The listing builds one solid part. Answer for the finished solid, in the listing's coordinates (mm). Face numbers are marked on the shaded views. A direction names the side the tool comes from. Give positions to 0.01 mm unless a question says otherwise; leave off trailing zeros. Write each loop counter-clockwise with the first axis right and the second up, starting at its lowest first coordinate (ties: lowest second). Pieces come first, ordered by that corner, then holes. Notation, with made-up numbers: (11, 47.25) - (22, 47.25) arc R20 cw to (22, 70.25) - close; hole circle Ø3 at (-14.75, 20.5). An arc over 180 degrees is marked (long way). Answer in a Markdown table with one row per item. Add a question column.
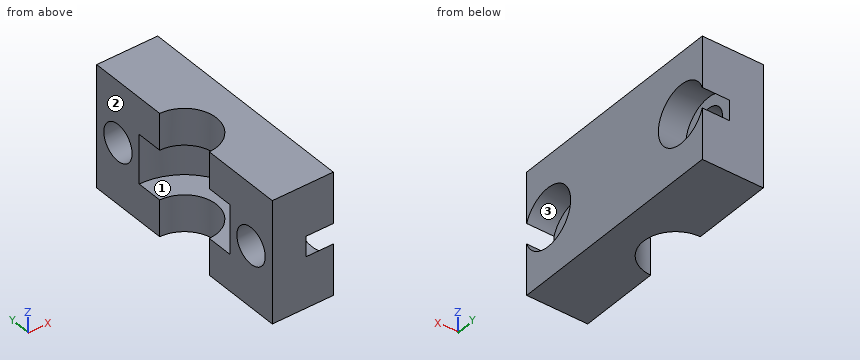
from build123d import *

# Parameters (mm, degrees)
EXTRUDE_1_DEPTH     = 2.7
SKETCH_1_4_W        = 3.35
SKETCH_1_4_H        = 12.4
EXTRUDE_2_DEPTH     = 2
EXTRUDE_START       = 2.7
SKETCH_1_5_W        = 3.35
SKETCH_1_5_H        = 12.4
EXTRUDE_3_DEPTH     = 2
SKETCH_2_R          = 1.75
CUT_EXTRUDE_1_DEPTH = 10.723810981
SKETCH_4_R          = 1
CUT_EXTRUDE_2_DEPTH = 9.470684742
SKETCH_4_3_R        = 1.6
SKETCH_4_3_R_2      = 1
CUT_EXTRUDE_3_DEPTH = 1.5


with BuildPart() as part:
    # 草图1 → 凸台-拉伸1 (new body)
    with BuildSketch(Plane.XY):
        with BuildLine():
            Line((3.35, 6.2), (0, 6.2))
            Line((0, 6.2), (0, 3.2))
            ThreePointArc((0, 3.2), (2.2627417, 2.2627417), (3.2, 0))
            ThreePointArc((3.2, 0), (2.2627417, -2.2627417), (0, -3.2))
            Line((0, -3.2), (0, -6.2))
            Line((0, -6.2), (3.35, -6.2))
            Line((3.35, -6.2), (3.35, 6.2))
        make_face()
    extrude(amount=EXTRUDE_1_DEPTH)

    # 草图1<4> → 凸台-拉伸2 (add)
    with BuildSketch(Plane.XY):
        with Locations((1.675, 0)):
            Rectangle(SKETCH_1_4_W, SKETCH_1_4_H)
    extrude(amount=-EXTRUDE_2_DEPTH)

    # 草图1<5> → 凸台-拉伸3 (add)
    with BuildSketch(Plane.XY.offset(EXTRUDE_START)):
        with Locations((1.675, 0)):
            Rectangle(SKETCH_1_5_W, SKETCH_1_5_H)
    extrude(amount=EXTRUDE_3_DEPTH)

    # 草图2 → 切除-拉伸1 (cut, through all)
    with BuildSketch(Plane.XY.offset(4.7)):
        Circle(SKETCH_2_R)
    extrude(amount=-CUT_EXTRUDE_1_DEPTH, mode=Mode.SUBTRACT)

    # 草图4 → 切除-拉伸2 (cut, through all)
    with BuildSketch(Plane(origin=(3.35, 0, 0), x_dir=(0, 0, -1), z_dir=(1, 0, 0))):
        with Locations((-1.35, -4.7)):
            Circle(SKETCH_4_R)
        with Locations((-1.35, 4.7)):
            Circle(SKETCH_4_R)
    extrude(amount=-CUT_EXTRUDE_2_DEPTH, mode=Mode.SUBTRACT)

    # 草图4<3> → 切除-拉伸3 (cut)
    # profile 1 of 2: a face of its own
    with BuildSketch(Plane(origin=(3.35, 0, 0), x_dir=(0, 0, -1), z_dir=(1, 0, 0))):
        with Locations((-1.35, 4.7)):
            Circle(SKETCH_4_3_R)
        with Locations((-1.35, 4.7)):
            Circle(SKETCH_4_3_R_2, mode=Mode.SUBTRACT)
    # profile 2 of 2: a face of its own
    with BuildSketch(Plane(origin=(3.35, 0, 0), x_dir=(0, 0, -1), z_dir=(1, 0, 0))):
        with Locations((-1.35, -4.7)):
            Circle(SKETCH_4_3_R)
        with Locations((-1.35, -4.7)):
            Circle(SKETCH_4_3_R_2, mode=Mode.SUBTRACT)
    extrude(amount=-CUT_EXTRUDE_3_DEPTH, mode=Mode.SUBTRACT)


solid = part.part
1. Straight lines are drawn through the part: L1, parallel to Z at x = 2.2, y = 0.5; L2, parallel to Y at x = 1, z = 1.35; L3, parallel to Y at x = 1.5, z = 0.5. For each, find the intervals that lie inside material, in ascending order. Write a range as [from, to].
2. Section C-C (y = 4.7) is taken. Give the vertices of the cut face in (x, z), and give its area (3 significant figures).
3. A tool of negligible diameter and unlimited length cuts with its end or side. For the marked faces 1, 2 and 3, from which of +Z, -Z, +X, -X, +Y, -Y can it reach the whole face along a straight path? Write none if from no direction.
4. Given pin 1 Ø2.5 at (y, z) = (-4.7, 1.35) entering from +X; pin 2 Ø3.5 at (y, z) = (-5, 2) entering from +X, each flat-ended and moving along its own axis, determine where each tip first touches the part or whether it passes through.
5. Section D-D (x = 2.25) is taken. Give the vertices of the cut face in (y, z).
6. Section B-B (x = 1.6) is taken. Give the vertices of the cut face in (y, z).
7. Section A-A (z = 1.35) is taken. Give the vertices of the cut face in (x, y).
Geometry check:
| question | item | result |
|---|---|---|
| 1 | L1 | [-2, 0], [2.7, 4.7] |
| 1 | L2 | [-6.2, -5.7], [-3.7, -3.04], [3.04, 3.7], [5.7, 6.2] |
| 1 | L3 | [-6.2, -5.23], [-4.17, -2.83], [2.83, 4.17], [5.23, 6.2] |
| 2 | outline | (0, -2) - (3.35, -2) - (3.35, -0.25) - (1.85, -0.25) - (1.85, 0.35) - (0, 0.35) - close; (0, 2.35) - (1.85, 2.35) - (1.85, 2.95) - (3.35, 2.95) - (3.35, 4.7) - (0, 4.7) - close |
| 2 | area | 13.9 mm² |
| 3 | face 1 | -X |
| 3 | face 2 | +Z, -Z, -X, +Y, -Y |
| 3 | face 3 | +X |
| 4 | pin 1 | x = 1.85 |
| 4 | pin 2 | x = 3.35 |
| 5 | outline | (-6.2, -2) - (6.2, -2) - (6.2, 0.79) arc R1.6 cw (long way) to (6.2, 1.91) - (6.2, 4.7) - (-6.2, 4.7) - (-6.2, 1.91) arc R1.6 cw (long way) to (-6.2, 0.79) - close; hole (-2.28, 0) - (2.28, 0) - (2.28, 2.7) - (-2.28, 2.7) - close |
| 6 | outline | (-6.2, -2) - (-0.71, -2) - (-0.71, 0) - (-2.77, 0) - (-2.77, 2.7) - (-0.71, 2.7) - (-0.71, 4.7) - (-6.2, 4.7) - close; (0.71, -2) - (6.2, -2) - (6.2, 4.7) - (0.71, 4.7) - (0.71, 2.7) - (2.77, 2.7) - (2.77, 0) - (0.71, 0) - close; hole circle Ø2 at (-4.7, 1.35); hole circle Ø2 at (4.7, 1.35) |
| 7 | outline | (0, -6.2) - (1.85, -6.2) - (1.85, -5.7) - (0, -5.7) - close; (0, -3.7) - (1.85, -3.7) - (1.85, -3.1) - (3.35, -3.1) - (3.35, 3.1) - (1.85, 3.1) - (1.85, 3.7) - (0, 3.7) - (0, 3.2) arc R3.2 cw to (0, -3.2) - close; (0, 5.7) - (1.85, 5.7) - (1.85, 6.2) - (0, 6.2) - close |
